The model under review builds one solid part; all positions refer to its coordinate system, in mm. Face numbers are marked on the shaded views. Give positions to 0.01 mm unless a question says otherwise; leave off trailing zeros. Loops run counter-clockwise (first coordinate to the right, second up) from the corner with the lowest first, then second, coordinate; pieces in that order, holes last. Notation, with made-up numbers: M -34.5,69.25 L -12.5,69.25 A29 cw -12.5,97.25 Z; hole C 11,79.5 d6. An arc over 180 degrees is marked long. Write item = value, one per line. Start each with the question number.
1. We need section B-B on y = 44.25. Give the boundary of the cut face in (x, z).
2. For pin 1 (2 mm diameter, centred on y = 46.5, z = 15, fed in from -X); pin 2 (3 mm diameter, centred on x = -0.5, y = 44.5, fed in from -Z); pin 3 (1.5 mm diameter, centred on y = 46, z = -20, fed in from -X), all flat-tipped, find the tip position at first contact; note any pin that passes through.
3. We need section A-A on x = 0. Give the boundary of the cut face in (y, z), then the cut area to 3 significant figures.
4. We need section D-D on z = 15. Give the boundary of the cut face in (x, y), then the cut area to 3 significant figures.
5. Wall thickness on line 1 along Z through (x, y) = (0, 42.75); line 2 along Y through (x, z) = (21, 9); line 3 along Z through (x, y) = (-24, 47.75): over which ranges is each line inside the solid? List them lowest first. Write a range as from..to.
6. We need section C-C on x = -23.75. Give the boundary of the cut face in (y, z), then the cut area to 3 significant figures.
7. Draft analysis for pull direction Z (two halves, no side actions). For the marked faces 1 and 2, state which applies: pulls with the +Z half, pulls with the -Z half, needs draft (parallel to the pull), parting line crosses it, or undercut.
Autodesk Inventor part; units mm, degrees
ref_plane "YZ Plane" through (0, 0, 0) normal (1, 0, 0) x (0, 1, 0)
ref_plane "XZ Plane" through (0, 0, 0) normal (0, 1, 0) x (-1, 0, 0)
ref_plane "XY Plane" through (0, 0, 0) normal (0, 0, 1) x (1, 0, 0)
sketch "Sketch1" plane through (0, 0, 0) normal (0, 1, 0) x (-1, 0, 0)
  circle A0 centre (0, 0) radius 28.5
  circle A1 centre (0, 0) radius 9
  circle A2 centre (11.875, 20.5681) radius 1.5875
  circle A3 centre (-11.875, 20.5681) radius 1.5875
  circle A4 centre (23.75, 0) radius 1.5875
  circle A5 centre (11.875, -20.5681) radius 1.5875
  circle A6 centre (-11.875, -20.5681) radius 1.5875
  circle A7 centre (-23.75, 0) radius 1.5875
  dimension "d5" = 3.175
  dimension "d6" = 20.5681
  dimension "d7" = 3.175
  dimension "d8" = 3.175
  dimension "d9" = 3.175
  dimension "d10" = 3.175
  dimension "d11" = 3.175
extrude "Extrusion1" add sketch "Sketch1" along normal blind 46
sketch "Sketch2" plane through (0, 46, 0) normal (0, 1, 0) x (1, 0, 0)
  line L0 (7.5157, 0) -> (3.7578, -6.5088)
  line L1 (3.7578, -6.5088) -> (-3.7578, -6.5088)
  line L2 (-3.7578, -6.5088) -> (-7.5157, 0)
  line L3 (-7.5157, 0) -> (-3.7578, 6.5088)
  line L4 (-3.7578, 6.5088) -> (3.7578, 6.5088)
  line L5 (3.7578, 6.5088) -> (7.5157, 0)
  circle A0 centre (0, 0) radius 28.5
  circle A1 centre (-11.875, -20.5681) radius 1.5875
  circle A2 centre (11.875, -20.5681) radius 1.5875
  circle A3 centre (-23.75, 0) radius 1.5875
  circle A4 centre (-11.875, 20.5681) radius 1.5875
  circle A5 centre (23.75, 0) radius 1.5875
  circle A6 centre (11.875, 20.5681) radius 1.5875
  dimension "d4" = 13.0175
extrude "Extrusion2" add sketch "Sketch2" against normal blind 46
sketch "Sketch3" plane through (0, 46, 0) normal (0, 1, 0) x (1, 0, 0)
  circle A0 centre (-11.875, 20.5681) radius 1.5875
  circle A1 centre (-11.875, 20.5681) radius 2.3812
  circle A2 centre (11.875, 20.5681) radius 1.5875
  circle A3 centre (11.875, 20.5681) radius 2.3812
  circle A4 centre (23.75, 0) radius 1.5875
  circle A5 centre (23.75, 0) radius 2.3813
  circle A6 centre (11.875, -20.5681) radius 1.5875
  circle A7 centre (11.875, -20.5681) radius 2.3813
  circle A8 centre (-11.875, -20.5681) radius 1.5875
  circle A9 centre (-11.875, -20.5681) radius 2.3812
  circle A10 centre (-23.75, 0) radius 1.5875
  circle A11 centre (-23.75, 0) radius 2.3812
  point P0 (0, 0)
  dimension "d12" = 4.7625
  dimension "d13" = 4.7625
  dimension "d14" = 4.7625
  dimension "d15" = 4.7625
  dimension "d16" = 4.7625
  dimension "d17" = 4.7625
extrude "Extrusion3" add sketch "Sketch3" along normal blind 2.3813 and the other way blind 48.3807 contours A0 | A1 | A2 | A3 | A4 | A5 | A6 | A7 | A8 | A9 | A10 | A11
sketch "Sketch4" plane through (11.875, -2.3806, 20.5681) normal (0, -1, 0) x (1, 0, 0)
  circle A0 centre (-11.875, -20.5681) radius 42.5802
extrude "Extrusion4" cut sketch "Sketch4" against normal blind 44.45
equation "\"d7\" = d5"
equation "\"d8\" = d5"
equation "\"d9\" = d5"
equation "\"d10\" = d5"
equation "\"d11\" = d5"
properties part number "2 thunder axel test v1"
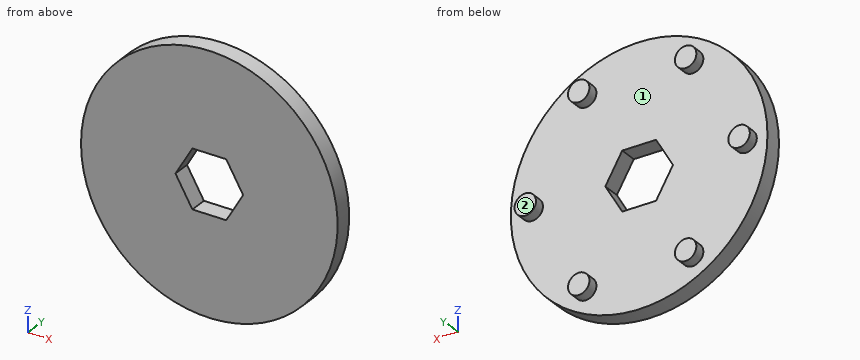
Final values:
q1.outline = C 0,0 d57; hole M -7.52,0 L -3.76,-6.51 L 3.76,-6.51 L 7.52,0 L 3.76,6.51 L -3.76,6.51 Z
q2.pin_1 = -24.75
q2.pin_2 = -28.5
q2.pin_3 = -21.02
q3.outline = M 42.07,-28.5 L 46,-28.5 L 46,-6.51 L 42.07,-6.51 Z; M 42.07,6.51 L 46,6.51 L 46,28.5 L 42.07,28.5 Z
q3.area = 173 mm²
q4.outline = M -24.23,42.07 L 24.23,42.07 L 24.23,46 L -24.23,46 Z
q4.area = 191 mm²
q5.line_1 = -28.5..-6.51, 6.51..28.5
q5.line_2 = 42.07..46
q5.line_3 = -2.37..2.37
q6.outline = M 42.07,-15.75 L 46,-15.75 L 46,-2.38 L 48.38,-2.38 L 48.38,2.38 L 46,2.38 L 46,15.75 L 42.07,15.75 Z
q6.area = 135 mm²
q7.face_1 = undercut
q7.face_2 = needs draft
